from build123d import *

# Parameters (mm, degrees)
SKETCH_1_W          = 256
SKETCH_1_H          = 70
EXTRUDE_1_DEPTH     = 4
FILLET_1_R          = 10
SHEET_START         = -128
SHEET_METAL_1_DEPTH = 256
FILLET_2_R          = 10


# Read off the part's stored shape, not the designer's step: Преобразовать-Твердое тело1
with BuildPart() as part:
    # Sketch 1 → Бобышка-Вытянуть1 (new, symmetric)
    with BuildSketch(Plane.XY):
        Rectangle(SKETCH_1_W, SKETCH_1_H)
    extrude(amount=EXTRUDE_1_DEPTH, both=True)

    # Скругление1
    # the kernel refuses this fillet: 10 mm, written as the material it takes off along each edge
    with BuildSketch(Plane(origin=(-152.494897428, -35, 4), x_dir=(0, 0, -1), z_dir=(1, 0, 0))) as fillet_1_piece_1:
        with BuildLine():
            CenterArc((10, 9.797958971), FILLET_1_R, 180, 78.463040967)
            Line((0, 9.797958971), (-0.2, 9.797958971))
            Line((-0.2, 9.797958971), (-0.2, 0))
            Line((-0.2, 0), (0, -0.2))
            ThreePointArc((0, -0.2), (4, -0.2), (7.96, -0.195959179))
            Line((7.96, -0.195959179), (8, 0))
        make_face()
    extrude(amount=304.989794856, mode=Mode.SUBTRACT)

    # Sheet Metal 1 outline → Sheet Metal 1 (add)
    with BuildSketch(Plane.YZ.offset(SHEET_START)):
        with BuildLine():
            Line((-35, 4), (-35, -4))
            ThreePointArc((-35, -4), (-31.526596349, 1.745966692), (-25.202041029, 4))
            Line((-25.202041029, 4), (-35, 4))
        make_face()
    extrude(amount=SHEET_METAL_1_DEPTH)

    # Скругление2
    # the kernel refuses this fillet: 10 mm, written as the material it takes off along each edge
    with BuildSketch(Plane(origin=(-152.494897428, -35, 4), x_dir=(0, 1, 0), z_dir=(1, 0, 0))) as fillet_2_piece_1:
        with BuildLine():
            CenterArc((9.797958971, -10), FILLET_2_R, 90, 78.463040967)
            Line((0, -8), (-0.195959179, -7.96))
            ThreePointArc((-0.195959179, -7.96), (-0.2, -4), (-0.2, 0))
            Line((-0.2, 0), (0, 0.2))
            Line((0, 0.2), (9.797958971, 0.2))
            Line((9.797958971, 0.2), (9.797958971, 0))
        make_face()
    extrude(amount=304.989794856, mode=Mode.SUBTRACT)

    # Эскиз8 → Зенковка для винта с потайной головкой M81 (revolve, cut)
    with BuildSketch(Plane(origin=(-68.5, -5, 4), x_dir=(0, -1, 0), z_dir=(1, 0, 0))):
        Polygon((0, 0), (0, 8), (4.5, 8), (4.5, 4.625), (9.125, 0), align=None)
    hole_wizard_m81 = revolve(axis=Axis((-68.5, -5, 10.35), (0, 0, -1)), mode=Mode.SUBTRACT)

    # Зеркальное отражение1: Зенковка для винта с потайной головкой M81 across plane
    add(hole_wizard_m81.mirror(Plane(origin=(0, 0, 0), x_dir=(0, 0, 1), z_dir=(1, 0, 0))), mode=Mode.SUBTRACT)


solid = part.part
Can you work these out from the model? Positions are in its coordinate system, mm. Round coordinates to 2 decimals unless told otherwise and drop trailing zeros. Write each loop counter-clockwise with the first axis right and the second up, starting at its lowest first coordinate (ties: lowest second). Pieces come first, ordered by that corner, then holes. Notation, with made-up numbers: M 24.25,-31.75 L 48.25,-31.75 A12 ccw 48.25,-27.75 Z; hole C -19,60.5 d2. An arc over 180 degrees is marked long. Use CSV: the item, a comma, the result in double quotes.
(1) Imagine slicing it at A-A (y = -5). Write out the boundary of the cut face in (x, z) (3 decimals), plus the area to 3 significant figures.
Check values:
outline,"M -128,-4 L -73,-4 L -73,-0.625 L -77.625,4 L -128,4 Z; M -64,-4 L 64,-4 L 64,-0.625 L 59.375,4 L -59.375,4 L -64,-0.625 Z; M 73,-4 L 128,-4 L 128,4 L 77.625,4 L 73,-0.625 Z"
area,"1,860 mm^2"
(2) We'd pull the mould along Y, two halves only. Please class faces 1 (the cylindrical face through (72.96, -4.41, -2.29)), 2 (the flat face through (-2, 35, 0)), 3 (the flat face through (-2, 5, 4)): +Y half, -Y half, draft (parallel to the pull), parting line (faces both ways), or undercut.
Check values:
face 1,"undercut"
face 2,"+Y half"
face 3,"draft"
(3) Imagine slicing it at C-C (z = 1.75). Write out the boundary of the cut face in (x, y) (3 decimals).
Check values:
outline,"M -128,-31.522 L 128,-31.522 L 128,35 L -128,35 Z; hole C -68.5,-5 d13.75; hole C 68.5,-5 d13.75"
(4) I'm going to push a flat-ended pin straight in: pin 1 (5.5 mm diameter, centred on x = 68.5, y = -5, fed in from -Z). Where does the tip first touch, or does it pass through?
Check values:
pin 1,"through"
(5) I need wall thicknesses on line 1 along X through (y, z) = (-5, -1.85); line 2 along X through (y, z) = (-3, 0); line 3 along Y through (x, z) = (-68.5, -2.5). Which ranges of each line are inside material? Lowest first, please.
Check values:
line 1,"-128 to -73, -64 to 64, 73 to 128"
line 2,"-128 to -73.22, -63.78 to 63.78, 73.22 to 128"
line 3,"-34.57 to -9.5, -0.5 to 35"
(6) Imagine slicing it at B-B (x = 68.5). Write out the boundary of the cut face in (y, z) (3 decimals), plus the area to 3 significant figures.
Check values:
outline,"M -35,-4 L -9.5,-4 L -9.5,-0.625 L -14.125,4 L -25.202,4 A10 ccw Z; M -0.5,-4 L 35,-4 L 35,4 L 4.125,4 L -0.5,-0.625 Z"
area,"447 mm^2"
(7) Imagine slicing it at D-D (x = -11.5). Write out the boundary of the cut face in (y, z).
Check values:
outline,"M -35,-4 L 35,-4 L 35,4 L -25.2,4 A10 ccw Z"
